For this review, take the finished solid that the model builds, in its own axes (mm). Face numbers are marked on the shaded views. A direction names the side the tool comes from. Coordinates: 2 decimals unless noted, no trailing zeros. Order: outer loops, then holes, each group sorted by start corner. A loop starts at its lowest first (then second) coordinate and runs counter-clockwise, first axis right, second up. Notation, with made-up numbers: (-9, 16.5) -> (4, 16.5) arc R12 cw to (4, 37.5) -> close; hole circle Ø5 at (16.5, 24.5). An arc over 180 degrees is marked (long way). Return JSON: item names as keys, results as strings. Group by question number.
Item 1: Machinability: for the marked faces 1 and 2, which of the approach directions +Z, -Z, +X, -X, +Y, -Y give a long, thin tool a straight path to every point of the face, cutting with its end or side? Answer none if there is none.
Item 2: Draft analysis for pull direction Y (two halves, no side actions). For the marked faces 3, 4 and 5, state which applies: +Y half, -Y half, draft (parallel to the pull), parting line (faces both ways), or undercut.
Item 3: Insertion check: pin 1 (8 mm diameter, centred on y = 8, z = 157.5, fed in from -X); pin 2 (7.5 mm diameter, centred on y = 29, z = 118, fed in from -X); pin 3 (12.5 mm diameter, centred on x = 19.5, z = 129, fed in from +Y). Each pin has a flat end and moves straight along its axis. Give the tip position at first contact, or say it passes through.
Item 4: Take a section at B-B (y = 32). Write out the cut boundary in (x, z).
Item 5: For line 1 along Y through (x, z) = (0, 109); line 2 along Y through (x, z) = (-20, 98), list the stretches that pass through material, from the lowest coordinate up.
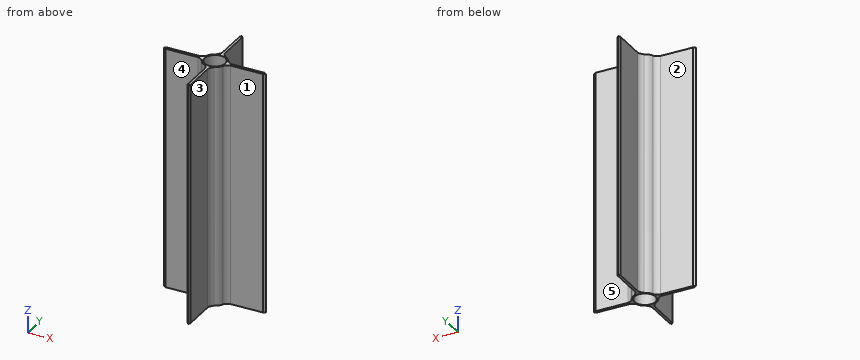
```python
from build123d import *

# Parameters (mm, degrees)
F0_R     = 8
F1_DEPTH = 185
F5_R     = 2
F6_DEPTH = 100


with BuildPart() as f1:
    # F0 (on Top) → F1 (new body)
    with BuildSketch(Plane.XY):
        with BuildLine():
            Line((-1, 37.4594671652), (-1, 12.4594671652))
            ThreePointArc((-1, 12.4594671652), (-1.9508662737, 10.095434036), (-3.6722679744, 8.2167175882))
            ThreePointArc((-3.6722679744, 8.2167175882), (-6.3639610307, 6.3639610307), (-8.2167175882, 3.6722679744))
            ThreePointArc((-8.2167175882, 3.6722679744), (-10.095434036, 1.9508662737), (-12.4594671652, 1))
            Line((-12.4594671652, 1), (-37.4594671652, 1))
            Line((-37.4594671652, 1), (-39, 0))
            Line((-39, 0), (-37.4594671652, -1))
            Line((-37.4594671652, -1), (-12.4594671652, -1))
            ThreePointArc((-12.4594671652, -1), (-10.095434036, -1.9508662737), (-8.2167175882, -3.6722679744))
            ThreePointArc((-8.2167175882, -3.6722679744), (-6.3639610307, -6.3639610307), (-3.6722679744, -8.2167175882))
            ThreePointArc((-3.6722679744, -8.2167175882), (-1.9508662737, -10.095434036), (-1, -12.4594671652))
            Line((-1, -12.4594671652), (-1, -37.4594671652))
            Line((-1, -37.4594671652), (0, -39))
            Line((0, -39), (1, -37.4594671652))
            Line((1, -37.4594671652), (1, -12.4594671652))
            ThreePointArc((1, -12.4594671652), (1.9508662737, -10.095434036), (3.6722679744, -8.2167175882))
            ThreePointArc((3.6722679744, -8.2167175882), (6.3639610307, -6.3639610307), (8.2167175882, -3.6722679744))
            ThreePointArc((8.2167175882, -3.6722679744), (10.095434036, -1.9508662737), (12.4594671652, -1))
            Line((12.4594671652, -1), (37.4594671652, -1))
            Line((37.4594671652, -1), (39, 0))
            Line((39, 0), (37.4594671652, 1))
            Line((37.4594671652, 1), (12.4594671652, 1))
            ThreePointArc((12.4594671652, 1), (10.095434036, 1.9508662737), (8.2167175882, 3.6722679744))
            ThreePointArc((8.2167175882, 3.6722679744), (6.3639610307, 6.3639610307), (3.6722679744, 8.2167175882))
            ThreePointArc((3.6722679744, 8.2167175882), (1.9508662737, 10.095434036), (1, 12.4594671652))
            Line((1, 12.4594671652), (1, 37.4594671652))
            Line((1, 37.4594671652), (0, 39))
            Line((0, 39), (-1, 37.4594671652))
        make_face()
        Circle(F0_R, mode=Mode.SUBTRACT)
    extrude(amount=F1_DEPTH)

    # F5 (on offset) → F6 (cut)
    with BuildSketch(Plane(origin=(-6.3639610307, -6.3639610307, 0), x_dir=(0.7071067812, -0.7071067812, 0), z_dir=(-0.7071067812, -0.7071067812, 0))):
        with Locations((0, 17.5)):
            Circle(F5_R)
        with Locations((0, 67.5)):
            Circle(F5_R)
        with Locations((0, 117.5)):
            Circle(F5_R)
        with Locations((0, 167.5)):
            Circle(F5_R)
    extrude(amount=-F6_DEPTH, mode=Mode.SUBTRACT)


solid = f1.part
```
Findings below:
{
 "1": {"face 1": "+Z, -Z, +X, -Y", "face 2": "+Z, -Z, -X, +Y"},
 "2": {"face 3": "draft", "face 4": "-Y half", "face 5": "+Y half"},
 "3": {"pin 1": "stops at x = -8.06", "pin 2": "stops at x = -1", "pin 3": "stops at y = 1"},
 "4": {"outline": "(-1, 0) -> (1, 0) -> (1, 185) -> (-1, 185) -> close"},
 "5": {"line 1": "y = -39 to -8, 8 to 39", "line 2": "y = -1 to 1"}
}
